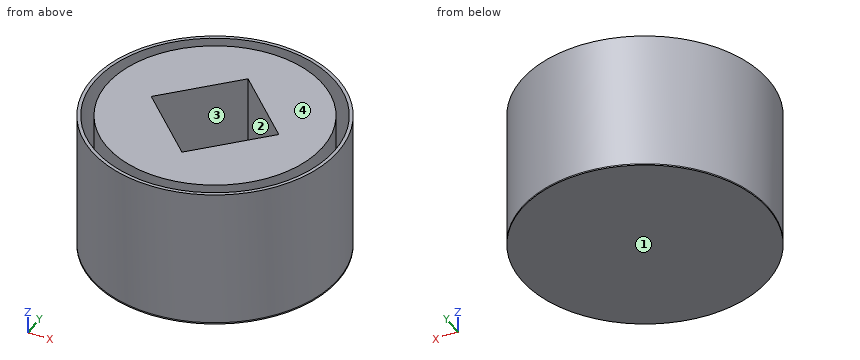
from build123d import *

# Parameters (mm, degrees)
F2_R     = 44.958
F3_DEPTH = 0.508
F4_R     = 39.37
F5_DEPTH = 50.8
F7_DEPTH = 33.02
F8_R     = 44.958
F8_R_2   = 43.688
F9_DEPTH = 50.8


# Not quite as in the source:
# - the program builds the solid bodies; features that only make, move or delete a surface that nothing else refers to are left out


with BuildPart() as f3:
    # F2 (on Top) → F3 (new body)
    with BuildSketch(Plane.XY):
        Circle(F2_R)
    extrude(amount=-F3_DEPTH)

    # F4 (on Top) → F5 (join)
    with BuildSketch(Plane.XY):
        Circle(F4_R)
    extrude(amount=F5_DEPTH)

    # F6 (on face) → F7 (cut)
    with BuildSketch(Plane.XY.offset(50.8)):
        Polygon((23.3486659148, 0), (0, 23.3486659148), (-23.3486659148, 0), (0, -23.3486659148), align=None)
    extrude(amount=-F7_DEPTH, mode=Mode.SUBTRACT)

    # F8 (on Top) → F9 (join)
    with BuildSketch(Plane.XY):
        Circle(F8_R)
        Circle(F8_R_2, mode=Mode.SUBTRACT)
    extrude(amount=F9_DEPTH)


solid = f3.part
Design review of the part built by this model. Coordinates are the model's own, in mm. Face numbers are marked on the shaded views. A direction names the side the tool comes from. Round coordinates to 2 decimals unless told otherwise and drop trailing zeros. Loops run counter-clockwise (first coordinate to the right, second up) from the corner with the lowest first, then second, coordinate; pieces in that order, holes last. Notation, with made-up numbers: (-12.5, 76.5) -> (22.5, 76.5) arc R24 cw to (22.5, 94.5) -> close; hole circle Ø8 at (58.5, 71). An arc over 180 degrees is marked (long way). Use one line per item in the form item = value. Start each with the question number.
Q1. We need section C-C on x = 16. Give the boundary of the cut face in (y, z), then the cut area to 3 significant figures.
Q2. We need section A-A on z = 41.5. Give the boundary of the cut face in (x, y).
Q3. Draft analysis for pull direction X (two halves, no side actions). For the marked faces 1 and 2, state which applies: +X half, -X half, draft (parallel to the pull), parting line (faces both ways), or undercut.
Q4. We need section D-D on y = 5. Give the boundary of the cut face in (x, z), then the cut area to 3 significant figures.
Q5. Machinability: for the marked faces 3 and 4, which of the approach directions +Z, -Z, +X, -X, +Y, -Y give a long, thin tool a straight path to every point of the face, cutting with its end or side? Answer none if there is none.
Q6. Wall thickness on line 1 along Y through (x, z) = (0, 20); line 2 along Y through (x, z) = (0, 16.5); line 3 along Y through (x, z) = (-10, 45): over which ranges is each line inside the solid? List them lowest first. Write a range as [from, to].
Q7. We need section B-B on z = 5.5. Give the boundary of the cut face in (x, y).
Q8. For pin 1 Ø1 at (y, z) = (-3.5, 35) entering from -X; pin 2 Ø8 at (x, z) = (18.5, 33) entering from -Y; pin 3 Ø1 at (y, z) = (-18, 6.5) entering from +X, all flat-tipped, find the tip position at first contact; note any pin that passes through.
Calculated:
q1.outline = (-42.01, -0.51) -> (42.01, -0.51) -> (42.01, 50.8) -> (40.65, 50.8) -> (40.65, 0) -> (35.97, 0) -> (35.97, 50.8) -> (7.35, 50.8) -> (7.35, 17.78) -> (-7.35, 17.78) -> (-7.35, 50.8) -> (-35.97, 50.8) -> (-35.97, 0) -> (-40.65, 0) -> (-40.65, 50.8) -> (-42.01, 50.8) -> close
q1.area = 3,350 mm²
q2.outline = circle Ø89.92 at (0, 0); circle Ø78.74 at (0, 0); hole circle Ø87.38 at (0, 0); hole (-23.35, 0) -> (0, -23.35) -> (23.35, 0) -> (0, 23.35) -> close
q3.face_1 = draft
q3.face_2 = undercut
q4.outline = (-44.68, -0.51) -> (44.68, -0.51) -> (44.68, 50.8) -> (43.4, 50.8) -> (43.4, 0) -> (39.05, 0) -> (39.05, 50.8) -> (18.35, 50.8) -> (18.35, 17.78) -> (-18.35, 17.78) -> (-18.35, 50.8) -> (-39.05, 50.8) -> (-39.05, 0) -> (-43.4, 0) -> (-43.4, 50.8) -> (-44.68, 50.8) -> close
q4.area = 2,930 mm²
q5.face_3 = +Z
q5.face_4 = +Z, +X, -X, +Y, -Y
q6.line_1 = [-44.96, -43.69], [-39.37, -23.35], [23.35, 39.37], [43.69, 44.96]
q6.line_2 = [-44.96, -43.69], [-39.37, 39.37], [43.69, 44.96]
q6.line_3 = [-43.83, -42.53], [-38.08, -13.35], [13.35, 38.08], [42.53, 43.83]
q7.outline = circle Ø89.92 at (0, 0); circle Ø78.74 at (0, 0); hole circle Ø87.38 at (0, 0)
q8.pin_1 = -44.86
q8.pin_2 = -42.56
q8.pin_3 = 41.41
